Job drawing, mm, ordinate dimensions from the low corner. One solid piece. Give positions to 0.01 mm unless a question says otherwise; leave off trailing zeros. Loops run counter-clockwise (first coordinate to the right, second up) from the corner with the lowest first, then second, coordinate; pieces in that order, holes last. Notation, with made-up numbers: (85.5, 69) - (99.5, 69) arc R21 ccw to (99.5, 75) - close; hole circle Ø9 at (-0.75, 89.5). An arc over 180 degrees is marked (long way). Use a Markdown table: item, result.
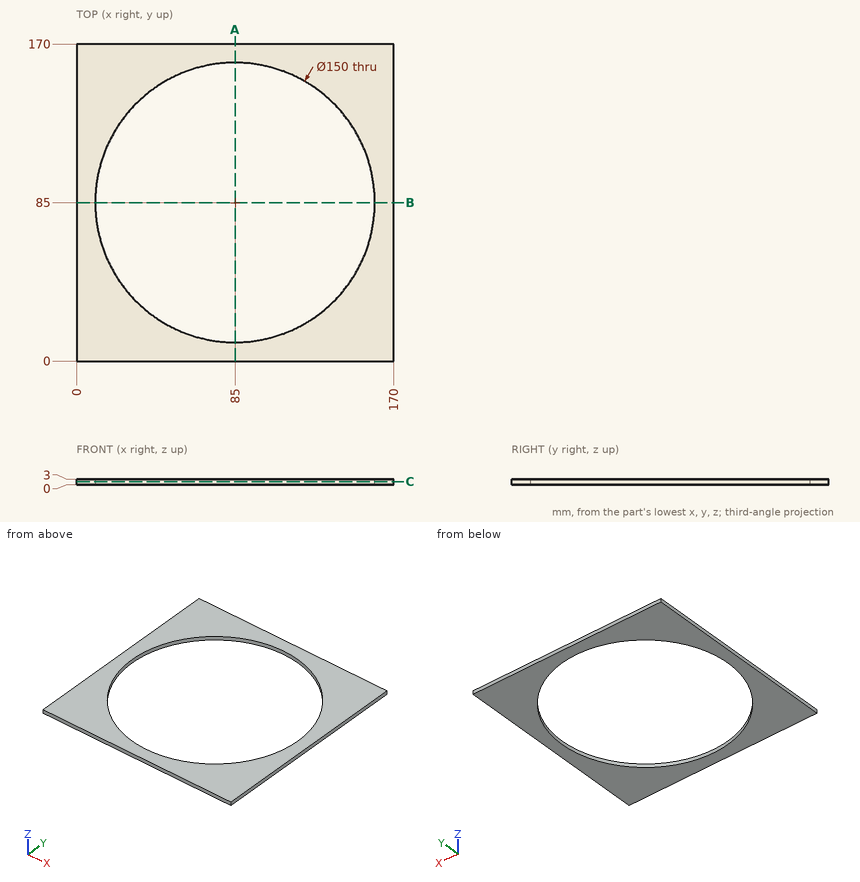
(1) Slice it at C-C, the plane z = 1.6. Write the cut outline in (x, y).
Computed:
| item | result |
|---|---|
| outline | (0, 0) - (170, 0) - (170, 170) - (0, 170) - close; hole circle Ø150 at (85, 85) |
(2) Drill centre lines: probe 1 along Y at (x, z) = (85, 1.65); probe 2 along Y at (x, z) = (33.5, 1.7); probe 3 along X at (y, z) = (100, 1.85). Where is each one in solid material? Low to high. Write a range as [from, to].
Computed:
| item | result |
|---|---|
| probe 1 | [0, 10], [160, 170] |
| probe 2 | [0, 30.48], [139.52, 170] |
| probe 3 | [0, 11.52], [158.48, 170] |
(3) Slice it at A-A, the plane x = 85. Write the cut outline in (y, z).
Computed:
| item | result |
|---|---|
| outline | (0, 0) - (10, 0) - (10, 3) - (0, 3) - close; (160, 0) - (170, 0) - (170, 3) - (160, 3) - close |
